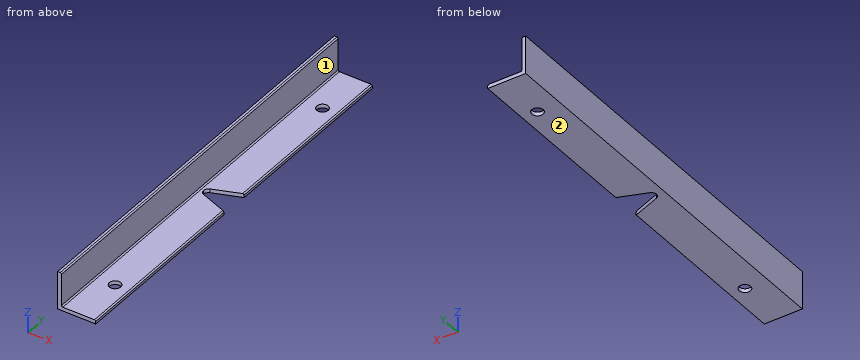
from build123d import *

# Parameters (mm, degrees)
F1_DEPTH = 320
F3_DEPTH = 30
F4_D     = 9


with BuildPart() as f1:
    # F0 (on Front) → F1 (new body)
    with BuildSketch(Plane.XZ):
        with BuildLine():
            Line((0, 30), (0, 0))
            Line((0, 0), (30, 0))
            Line((30, 0), (30, 2))
            ThreePointArc((30, 2), (29.7071067812, 2.7071067812), (29, 3))
            Line((29, 3), (4, 3))
            ThreePointArc((4, 3), (3.2928932188, 3.2928932188), (3, 4))
            Line((3, 4), (3, 29))
            ThreePointArc((3, 29), (2.7071067812, 29.7071067812), (2, 30))
            Line((2, 30), (0, 30))
        make_face()
    extrude(amount=F1_DEPTH)

    # F2 (on Top) → F3 (cut, through all)
    with BuildSketch(Plane.XY):
        with BuildLine():
            Line((30, -148.180951785), (8.5882981113, -156.257394253))
            ThreePointArc((8.5882981113, -156.257394253), (6.7101058106, -157.7247865545), (6, -160))
            ThreePointArc((6, -160), (6.7101058106, -162.2752134455), (8.5882981113, -163.742605747))
            Line((8.5882981113, -163.742605747), (30, -171.819048215))
            Line((30, -171.819048215), (30, -160))
            Line((30, -160), (30, -148.180951785))
        make_face()
    extrude(amount=F3_DEPTH, mode=Mode.SUBTRACT)

    # F4 (through all)
    with Locations(Plane(origin=(0, 0, 0), x_dir=(1, 0, 0), z_dir=(0, 0, -1))):
        with Locations((18, 40), (18, 280)):
            Hole(F4_D / 2)


solid = f1.part
The model under review builds one solid part; all positions refer to its coordinate system, in mm. Face numbers are marked on the shaded views. A direction names the side the tool comes from. Give positions to 0.01 mm unless a question says otherwise; leave off trailing zeros. Loops run counter-clockwise (first coordinate to the right, second up) from the corner with the lowest first, then second, coordinate; pieces in that order, holes last. Notation, with made-up numbers: (65.5, 44.25) -> (119.5, 44.25) arc R24 ccw to (119.5, 62.25) -> close; hole circle Ø2 at (69, 72). An arc over 180 degrees is marked (long way). Answer as a JSON object with one key per item and string values. Group by question number.
Q1. Wall thickness on line 1 along X through (y, z) = (-280, 1.15); line 2 along X through (y, z) = (-130.5, 15.5); line 3 along Y through (x, z) = (18, 1.75): over which ranges is each line inside the solid? List them lowest first.
Q2. Take a section at B-B (x = 18). Write out the cut boundary in (y, z).
Q3. Take a section at C-C (z = 8). Write out the cut boundary in (x, y).
Q4. Tool access review of the marked faces 1 and 2: name each direction out of +Z, -Z, +X, -X, +Y, -Y from which nothing blocks a thin tool from reaching the whole face with its end or side.
Q5. Insertion check: pin 1 (2 mm diameter, centred on x = 19.5, y = -49, fed in from -Z); pin 2 (12 mm diameter, centred on y = -38.5, z = 14.5, fed in from +X); pin 3 (12.5 mm diameter, centred on x = 13.5, y = -109.5, fed in from +Z); pin 4 (7 mm diameter, centred on x = 18, y = -40, fed in from -Z). Each pin has a flat end and moves straight along its axis. Give the tip position at first contact, or say it passes through.
Q6. Take a section at A-A (y = -280). Write out the cut boundary in (x, z).
Answer below:
{
 "1": {"line 1": "x = 0 to 13.5, 22.5 to 30", "line 2": "x = 0 to 3", "line 3": "y = -320 to -284.5, -275.5 to -167.29, -152.71 to -44.5, -35.5 to 0"},
 "2": {"outline": "(-320, 0) -> (-284.5, 0) -> (-284.5, 3) -> (-320, 3) -> close; (-275.5, 0) -> (-167.29, 0) -> (-167.29, 3) -> (-275.5, 3) -> close; (-152.71, 0) -> (-44.5, 0) -> (-44.5, 3) -> (-152.71, 3) -> close; (-35.5, 0) -> (0, 0) -> (0, 3) -> (-35.5, 3) -> close"},
 "3": {"outline": "(0, -320) -> (3, -320) -> (3, 0) -> (0, 0) -> close"},
 "4": {"face 1": "+Z, +X, +Y, -Y", "face 2": "-Z, +X, -X, +Y, -Y"},
 "5": {"pin 1": "stops at z = 0", "pin 2": "stops at x = 3", "pin 3": "stops at z = 3", "pin 4": "passes through"},
 "6": {"outline": "(0, 0) -> (13.5, 0) -> (13.5, 3) -> (4, 3) arc R1 cw to (3, 4) -> (3, 29) arc R1 ccw to (2, 30) -> (0, 30) -> close; (22.5, 0) -> (30, 0) -> (30, 2) arc R1 ccw to (29, 3) -> (22.5, 3) -> close"}
}
